Model file for the job. Use its own axes, mm. A direction names the side the tool comes from. Round coordinates to 2 decimals unless told otherwise and drop trailing zeros. Loops run counter-clockwise (first coordinate to the right, second up) from the corner with the lowest first, then second, coordinate; pieces in that order, holes last. Notation, with made-up numbers: M 74.25,-19 L 112.25,-19 A4 ccw 112.25,-12 Z; hole C -24,76 d8. An arc over 180 degrees is marked long. Use a Markdown table: item, result. Add a question column.
Item 1: Saw through at B-B on y = 7. Write the cut outline in (x, z).
Item 2: Saw through at D-D on z = -62. Write the cut outline in (x, y), then the cut area to 3 significant figures.
Item 3: Saw through at A-A on x = 2.45. Write the cut outline in (y, z), then the cut area to 3 significant figures.
Item 4: Tool access for faces 5 (the cylindrical face through (1.48, -1.27, -0.97)), 6 (the flat face through (1, 13, -76)): list every direction of +Z, -Z, +X, -X, +Y, -Y with a clear straight run to the whole face (end or side of a thin tool).
Item 5: Saw through at C-C on z = -7. Write the cut outline in (x, y).
Item 6: Wall check: L1, parallel to Z at x = 0.7, y = -0.5; L2, parallel to Z at x = 2.45, y = -7.5; L3, parallel to Y at x = 2.05, z = -77. Give the ranges that are in metal, low to high. Write a range as from..to.
Item 7: Two-plate mould, pull along Y, no slides. Class faces 1 (the cylindrical face through (1.479, 17.155, -103.807)), 2 (the cylindrical face through (1.521, 12.626, -93.695)), 3 (the flat face through (1.48, 15.55, -13.49)), 4 (the flat face through (3, 11, -35)): +Y half, -Y half, draft (parallel to the pull), parting line (faces both ways), or undercut.
Item 8: Pin check, flat tip, straight feed: P1, Ø1, axis at x = 2, z = -34.5, coming from the +Y side. Stop position of the tip, or through.
```python
from build123d import *

# Parameters (mm, degrees)
SKETCH049_R   = 1.6
SKETCH049_R_2 = 3.9
PAD027_DEPTH  = 3
FILLET016_R   = 60
FILLET017_R   = 10


with BuildPart() as part:
    # Sketch049 → Pad027 (new body)
    with BuildSketch(Plane.YZ):
        with BuildLine():
            ThreePointArc((9.3969262079, 3.4202014333), (-7.6604444312, 6.4278760969), (-1.7364817767, -9.8480775301))
            Line((-1.7364817767, -9.8480775301), (13, -50.3362284537))
            Line((13, -50.3362284537), (13, -94.4098300562))
            ThreePointArc((13, -94.4098300562), (14.9381378215, -106.8465319688), (25.5, -100))
            Line((25.5, -40.8226301945), (25.5, -100))
            Line((9.3969262079, 3.4202014333), (25.5, -40.8226301945))
        make_face()
        with Locations((0, 7)):
            Circle(SKETCH049_R, mode=Mode.SUBTRACT)
        with Locations((7, 0)):
            Circle(SKETCH049_R, mode=Mode.SUBTRACT)
        with Locations((0, -7)):
            Circle(SKETCH049_R, mode=Mode.SUBTRACT)
        with Locations((-7, 0)):
            Circle(SKETCH049_R, mode=Mode.SUBTRACT)
        Circle(SKETCH049_R, mode=Mode.SUBTRACT)
        with Locations((18, -100)):
            Circle(SKETCH049_R_2, mode=Mode.SUBTRACT)
    extrude(amount=PAD027_DEPTH)

    # Fillet016
    fillet016_edges = [part.edges().sort_by_distance(p)[0] for p in [
        (1.5, 13, -50.336228),
        (1.5, 25.5, -40.82263),
    ]]
    fillet(fillet016_edges, radius=FILLET016_R)

    # Fillet017
    fillet017_edges = [part.edges().sort_by_distance(p)[0] for p in [
        (1.5, 13, -94.40983),
        (1.5, -1.736482, -9.848078),
    ]]
    fillet(fillet017_edges, radius=FILLET017_R)


solid = part.part
```
Entries:
| question | item | result |
|---|---|---|
| 1 | outline | M 0,-33.85 L 3,-33.85 L 3,-1.6 L 0,-1.6 Z; M 0,1.6 L 3,1.6 L 3,7.14 L 0,7.14 Z |
| 2 | outline | M 0,13 L 3,13 L 3,25.5 L 0,25.5 Z |
| 2 | area | 37.5 mm2 |
| 3 | outline | M -4.79,-8.78 A10 cw -0.17,-14.14 L 9.38,-40.39 A60 cw 13,-60.92 L 13,-90.99 A10 cw 11.57,-96.14 A7.5 ccw long 25.5,-100 L 25.5,-51.4 A60 ccw 21.88,-30.88 L 9.4,3.42 A10 ccw long Z; hole C -7,0 d3.2; hole C 0,-7 d3.2; hole C 0,0 d3.2; hole C 0,7 d3.2; hole C 7,0 d3.2; hole C 18,-100 d7.8 |
| 3 | area | 1,620 mm2 |
| 4 | face 5 | +X, -X |
| 4 | face 6 | +X, -X, -Y |
| 5 | outline | M 0,-7.14 L 3,-7.14 L 3,-1.6 L 0,-1.6 Z; M 0,1.6 L 3,1.6 L 3,13.19 L 0,13.19 Z |
| 6 | L1 | -13.35..-8.52, -5.48..-1.52, 1.52..5.48, 8.52..9.99 |
| 6 | L2 | -6.61..-1.52, 1.52..6.61 |
| 6 | L3 | 13..25.5 |
| 7 | face 1 | undercut |
| 7 | face 2 | -Y half |
| 7 | face 3 | +Y half |
| 7 | face 4 | draft |
| 8 | P1 | y = 23.21 |
